Could you check a few things on this model? Use its own coordinates, in mm. Face numbers are marked on the shaded views. A direction names the side the tool comes from. Coordinates: 2 decimals unless noted, no trailing zeros. Order: outer loops, then holes, each group sorted by start corner. A loop starts at its lowest first (then second) coordinate and runs counter-clockwise, first axis right, second up.
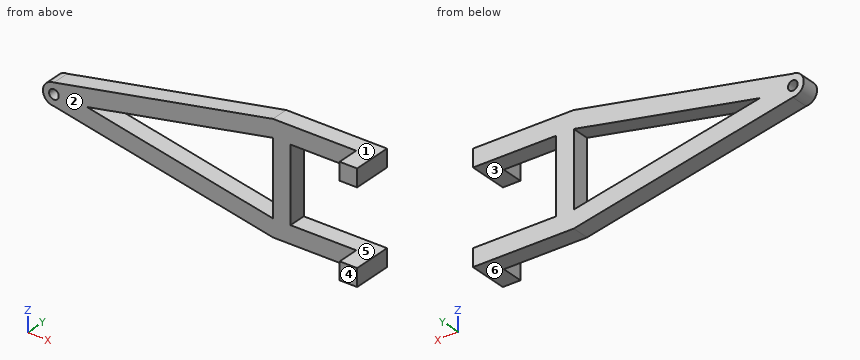
```python
from build123d import *

# Parameters (mm, degrees)
SKETCH1_W           = 4
SKETCH1_H           = 25
SKETCH1_W_2         = 19
SKETCH1_H_2         = 4
SKETCH1_R           = 2.5
SKETCH1_R_2         = 1.1
BOSS_EXTRUDE1_DEPTH = 4
SKETCH2_W           = 4
SKETCH2_H           = 4
BOSS_EXTRUDE2_DEPTH = 5


with BuildPart() as part:
    # Sketch1 → Boss-Extrude1 (new body)
    # profile 1 of 7: a face of its own
    with BuildSketch(Plane(origin=(0, 0, 0), x_dir=(1, 0, 0), z_dir=(0, 1, 0))):
        with BuildLine():
            Line((15.760200843, 53.402286132), (-34.239799157, 43.402286132))
            ThreePointArc((-34.239799157, 43.402286132), (-32.891585166, 43.007593481), (-31.969075298, 41.94814136))
            Line((-31.969075298, 41.94814136), (-26.739799157, 40.902286132))
            Line((-26.739799157, 40.902286132), (15.760200843, 49.402286132))
            Line((15.760200843, 49.402286132), (15.760200843, 53.402286132))
        make_face()
    # profile 2 of 7: a face of its own
    with BuildSketch(Plane(origin=(0, 0, 0), x_dir=(1, 0, 0), z_dir=(0, 1, 0))):
        with Locations((17.760200843, 40.902286132)):
            Rectangle(SKETCH1_W, SKETCH1_H)
    # profile 3 of 7: a face of its own
    with BuildSketch(Plane(origin=(0, 0, 0), x_dir=(1, 0, 0), z_dir=(0, 1, 0))):
        with Locations((29.260200843, 51.402286132)):
            Rectangle(SKETCH1_W_2, SKETCH1_H_2)
    # profile 4 of 7: a face of its own
    with BuildSketch(Plane(origin=(0, 0, 0), x_dir=(1, 0, 0), z_dir=(0, 1, 0))):
        with Locations((29.260200843, 30.402286132)):
            Rectangle(SKETCH1_W_2, SKETCH1_H_2)
    # profile 5 of 7: a face of its own
    with BuildSketch(Plane(origin=(0, 0, 0), x_dir=(1, 0, 0), z_dir=(0, 1, 0))):
        with BuildLine():
            Line((-26.739799157, 40.902286132), (-31.969075298, 41.94814136))
            ThreePointArc((-31.969075298, 41.94814136), (-31.797790798, 41.43763198), (-31.739799157, 40.902286132))
            ThreePointArc((-31.739799157, 40.902286132), (-31.797790798, 40.366940284), (-31.969075298, 39.856430904))
            Line((-31.969075298, 39.856430904), (-26.739799157, 40.902286132))
        make_face()
    # profile 6 of 7: a face of its own
    with BuildSketch(Plane(origin=(0, 0, 0), x_dir=(1, 0, 0), z_dir=(0, 1, 0))):
        with Locations((-34.239799157, 40.902286132)):
            Circle(SKETCH1_R)
        with Locations(Location((-34.239799157, 40.902286132, 0), (0, 0, 270))):
            Circle(SKETCH1_R_2, mode=Mode.SUBTRACT)
    # profile 7 of 7: a face of its own
    with BuildSketch(Plane(origin=(0, 0, 0), x_dir=(1, 0, 0), z_dir=(0, 1, 0))):
        with BuildLine():
            ThreePointArc((-31.969075298, 39.856430904), (-32.891585166, 38.796978783), (-34.239799157, 38.402286132))
            Line((-34.239799157, 38.402286132), (15.760200843, 28.402286132))
            Line((15.760200843, 28.402286132), (15.760200843, 32.402286132))
            Line((15.760200843, 32.402286132), (-26.739799157, 40.902286132))
            Line((-26.739799157, 40.902286132), (-31.969075298, 39.856430904))
        make_face()
    extrude(amount=BOSS_EXTRUDE1_DEPTH)

    # Sketch2 → Boss-Extrude2 (add)
    with BuildSketch(Plane.XZ):
        with Locations((36.760200843, -30.402286132)):
            Rectangle(SKETCH2_W, SKETCH2_H)
        with Locations((36.760200843, -51.402286132)):
            Rectangle(SKETCH2_W, SKETCH2_H)
    extrude(amount=BOSS_EXTRUDE2_DEPTH)


solid = part.part
```
Item 1: Suppose I cut it at C-C (x = -8.5). List the corners of the cut face in (y, z) for me.
Item 2: Suppose I cut it at B-B (y = 2). List the corners of the cut face in (x, z) for me.
Item 3: Suppose I cut it at D-D (x = 17). List the corners of the cut face in (y, z) for me.
Item 4: Thinking about a two-plate mould opening in Z: for the marked faces 4, 5 and 6, which applies, +Z half, -Z half, draft (parallel to the pull), parting line (faces both ways), or undercut?
Item 5: For pin 1 Ø4.5 at (y, z) = (-2.5, -31) entering from -X; pin 2 Ø4.5 at (y, z) = (2.5, -39) entering from +X; pin 3 Ø4.5 at (y, z) = (1, -45) entering from -X, each with a flat end and sliding along its axis, tell me the tip position at first contact or that it passes through.
Item 6: I need wall thicknesses on line 1 (Z direction, x = 27, y = 0.75); line 2 (Z direction, x = 1.5, y = 0.5); line 3 (Y direction, x = 18.5, z = -47). Which ranges of each line are inside material? Lowest first, please.
Item 7: Which directions (+Z, -Z, +X, -X, +Y, -Y) give clear straight access to the entire face, cutting with the end or side of a thin tool? Please do the marked faces 1, 2 and 3.
Item 8: Suppose I cut it at A-A (y = -3.5). List the corners of the cut face in (x, z) for me.
Geometry results:
1. outline: (0, -48.55) - (4, -48.55) - (4, -44.55) - (0, -44.55) - close; (0, -37.25) - (4, -37.25) - (4, -33.25) - (0, -33.25) - close
2. outline: (-34.24, -43.4) - (15.76, -53.4) - (38.76, -53.4) - (38.76, -49.4) - (19.76, -49.4) - (19.76, -32.4) - (38.76, -32.4) - (38.76, -28.4) - (15.76, -28.4) - (-34.24, -38.4) arc R2.5 ccw to start; hole circle Ø2.2 at (-34.24, -40.9); hole (-26.74, -40.9) - (15.76, -49.4) - (15.76, -32.4) - close
3. outline: (0, -53.4) - (4, -53.4) - (4, -28.4) - (0, -28.4) - close
4. face 4: draft
4. face 5: undercut
4. face 6: -Z half
5. pin 1: stops at x = 34.76
5. pin 2: stops at x = 19.76
5. pin 3: stops at x = -35.92
6. line 1: z = -53.4 to -49.4, -32.4 to -28.4
6. line 2: z = -50.55 to -46.55, -35.25 to -31.25
6. line 3: y = 0 to 4
7. face 1: +Z, +X, -X, +Y, -Y
7. face 2: +Z, -Z, -X, -Y
7. face 3: +X, +Y, -Y
8. outline: (34.76, -53.4) - (38.76, -53.4) - (38.76, -49.4) - (34.76, -49.4) - close; (34.76, -32.4) - (38.76, -32.4) - (38.76, -28.4) - (34.76, -28.4) - close
